from build123d import *

# Parameters (mm, degrees)
SKETCH1_W           = 10
SKETCH1_H           = 3
BOSS_EXTRUDE1_DEPTH = 0.5
BOSS_EXTRUDE2_DEPTH = 3
CUT_EXTRUDE1_REACH  = 9.27
SKETCH4_R           = 1.5
CUT_EXTRUDE2_REACH  = 9.12
SKETCH5_R           = 0.5


with BuildPart() as part:
    # Sketch1 → Boss-Extrude1 (new, symmetric)
    with BuildSketch(Plane(origin=(0, 0, 0), x_dir=(1, 0, 0), z_dir=(0, 1, 0))):
        Rectangle(SKETCH1_W, SKETCH1_H)
    extrude(amount=BOSS_EXTRUDE1_DEPTH, both=True)

    # Sketch3 → Boss-Extrude2 (add)
    with BuildSketch(Plane(origin=(0, 0, -1.5), x_dir=(-1, 0, 0), z_dir=(0, 0, -1))):
        with BuildLine():
            Line((-5, 0.5), (-5, 0))
            Line((-5, 0), (5, 0))
            Line((5, 0), (5, 0.5))
            ThreePointArc((5, 0.5), (3.589234213, 0.859934084), (2.514072517, 1.841687605))
            ThreePointArc((2.514072517, 1.841687605), (0.014072517, 4.341687605), (-2.485927483, 1.841687605))
            ThreePointArc((-2.485927483, 1.841687605), (-3.573488857, 0.853279454), (-5, 0.5))
        make_face()
    extrude(amount=-BOSS_EXTRUDE2_DEPTH)

    # Sketch4 → Cut-Extrude1 (cut, up to next)
    with BuildSketch(Plane(origin=(0, 0, -1.5), x_dir=(-1, 0, 0), z_dir=(0, 0, -1)), mode=Mode.PRIVATE) as cut_extrude1_sk1:
        with Locations((0.014072517, 1.841687605)):
            Circle(SKETCH4_R)
    cut_extrude1_tool1 = extrude(cut_extrude1_sk1.sketch, amount=-CUT_EXTRUDE1_REACH, mode=Mode.PRIVATE) & part.part
    add(cut_extrude1_tool1.solids().sort_by_distance((-0.014073, 1.841688, -1.5))[0], mode=Mode.SUBTRACT)

    # Sketch5 → Cut-Extrude2 (cut, up to next)
    with BuildSketch(Plane.XZ.offset(0.5), mode=Mode.PRIVATE) as cut_extrude2_sk1:
        with Locations(Location((-4, 0, 0), (0, 0, 270))):
            Circle(SKETCH5_R)
    cut_extrude2_tool1 = extrude(cut_extrude2_sk1.sketch, amount=-CUT_EXTRUDE2_REACH, mode=Mode.PRIVATE) & part.part
    # Sketch5 → Cut-Extrude2 (cut, up to next)
    with BuildSketch(Plane.XZ.offset(0.5), mode=Mode.PRIVATE) as cut_extrude2_sk2:
        with Locations(Location((4, 0, 0), (0, 0, 270))):
            Circle(SKETCH5_R)
    cut_extrude2_tool2 = extrude(cut_extrude2_sk2.sketch, amount=-CUT_EXTRUDE2_REACH, mode=Mode.PRIVATE) & part.part
    add(cut_extrude2_tool1.solids().sort_by_distance((-4, -0.5, 0))[0], mode=Mode.SUBTRACT)
    add(cut_extrude2_tool2.solids().sort_by_distance((4, -0.5, 0))[0], mode=Mode.SUBTRACT)


solid = part.part
Source: CAD feature listing. Evaluate the final solid. Frame: model axes, mm. Give positions to 0.01 mm unless a question says otherwise; leave off trailing zeros. Write each loop counter-clockwise with the first axis right and the second up, starting at its lowest first coordinate (ties: lowest second). Pieces come first, ordered by that corner, then holes. Notation, with made-up numbers: (-11, 35.25) -> (3, 35.25) arc R24 ccw to (3, 66.25) -> close; hole circle Ø11 at (68.5, 32.25). An arc over 180 degrees is marked (long way). Return JSON: item names as keys, results as strings. Group by question number.
1. Material intervals for line 1 (X direction, y = -0.2, z = 0); line 2 (X direction, y = 1.9, z = 0.9); line 3 (Z direction, x = 4, y = -0.2), sorted ascending. Write a range as from..to.
2. Mould query, pull axis X, two halves, no side actions, for faces 1 (the face through (-3.504, 0.038, 0.065)), 2 (the face through (5, 0, 0)), 3 (the face through (0, 0, 1.5)), 4 (the face through (-3.328, 1.019, -0.021)). Classes: +X half, -X half, draft (parallel to the pull), parting line (faces both ways), or undercut.
3. Section B-B, the plane x = -4. Output: boundary loops of the cut face in (y, z), then the cut area to 3 significant figures.
4. Section D-D, the plane y = 2.85. Output: boundary loops of the cut face in (x, z).
5. Section A-A, the plane z = 0.15. Count the separate pieces of the cut face and the enclosed holes in it, then the cut area to 3 significant figures.
Determined:
{
 "1": {"line 1": "x = -5..-4.5, -3.5..3.5, 4.5..5", "line 2": "x = -2.51..-1.51, 1.48..2.49", "line 3": "z = -1.5..-0.5, 0.5..1.5"},
 "2": {"face 1": "undercut", "face 2": "+X half", "face 3": "draft", "face 4": "-X half"},
 "3": {"outline": "(-0.5, -1.5) -> (0.68, -1.5) -> (0.68, -0.5) -> (-0.5, -0.5) -> close; (-0.5, 0.5) -> (0.68, 0.5) -> (0.68, 1.5) -> (-0.5, 1.5) -> close", "area": "2.35 mm2"},
 "4": {"outline": "(-2.3, -1.5) -> (-1.12, -1.5) -> (-1.12, 1.5) -> (-2.3, 1.5) -> close; (1.1, -1.5) -> (2.27, -1.5) -> (2.27, 1.5) -> (1.1, 1.5) -> close"},
 "5": {"separate pieces": "3", "enclosed holes": "1", "area": "19.2 mm2"}
}
